from build123d import *

# Parameters (mm, degrees)
SKETCH_5_R = 7.5


with BuildPart() as part:
    # По траектории3: sweep along a path in Эскиз4
    with BuildLine(Plane.XY) as sweep_3_path:
        Line((-180, -170), (-120, -170))
        ThreePointArc((-120, -170), (-70.502525317, -149.497474683), (-50, -100))
        Line((-50, -100), (-50, -50))
        ThreePointArc((-50, -50), (-35.355339059, -14.644660941), (0, 0))
    # Эскиз5 → По траектории3 (sweep)
    with BuildSketch(Plane(origin=(0, 0, 0), x_dir=(0, 0, -1), z_dir=(1, 0, 0))):
        Circle(SKETCH_5_R)
    sweep_3 = sweep(path=sweep_3_path.line)

    # Зеркальное отражение4: По траектории3 across plane
    add(sweep_3.mirror(Plane(origin=(0, 0, 0), x_dir=(0, 0, 1), z_dir=(1, 0, 0))))


solid = part.part
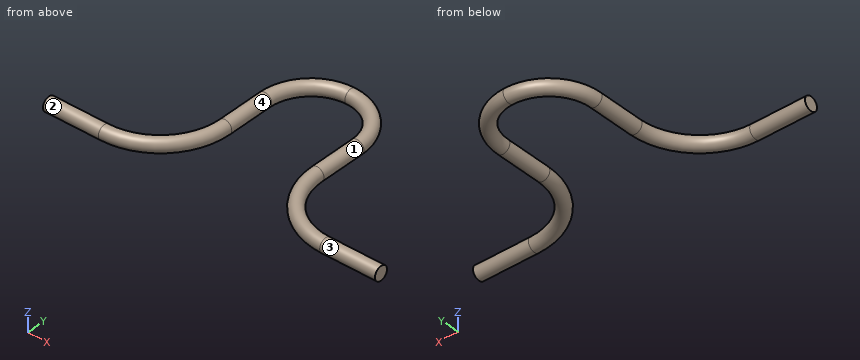
Can you work these out from the model? Positions are in its coordinate system, mm. Face numbers are marked on the shaded views. A direction names the side the tool comes from. Round coordinates to 2 decimals unless told otherwise and drop trailing zeros. Loops run counter-clockwise (first coordinate to the right, second up) from the corner with the lowest first, then second, coordinate; pieces in that order, holes last. Notation, with made-up numbers: (-23.75, 23) - (-13.75, 23) arc R24 cw to (-13.75, 39) - close; hole circle Ø9 at (-9.75, 18.25). An arc over 180 degrees is marked (long way). Answer in a Markdown table with one row per item. Add a question column.
Q1. We'd pull the mould along X, two halves only. Please class the marked faces 1 and 2: pulls with the +X half, pulls with the -X half, needs draft (parallel to the pull), parting line crosses it, or undercut.
Q2. I need wall thicknesses on L1, parallel to X at y = -52, z = 1; L2, parallel to X at y = -12, z = -0.5; L3, parallel to Y at x = -136, z = -0.5. Which ranges of each line are inside material? Lowest first, please.
Q3. I want a section at B-B on y = -66. List the corners of the cut face in (x, z) for me, and give its area (3 significant figures).
Q4. Which directions (+Z, -Z, +X, -X, +Y, -Y) give clear straight access to the entire face, cutting with the end or side of a thin tool? Please do the marked faces 3 and 4.
Q5. For pin 1 Ø5 at (y, z) = (-43.5, 5.5) entering from +X; pin 2 Ø3 at (x, z) = (79, -4.5) entering from -Y; pin 3 Ø1 at (x, z) = (-116, 1) entering from +Y, each with a flat end and sliding along its axis, tell me the tip position at first contact or that it passes through.
Q6. I want a section at A-A on z = 0. List the corners of the cut face in (x, y) for me.
Q7. I want a section at C-C on x = -131. List the corners of the cut face in (y, z) for me.
A:
| question | item | result |
|---|---|---|
| 1 | face 1 | undercut |
| 1 | face 2 | needs draft |
| 2 | L1 | -57.43 to -42.57, 42.57 to 57.43 |
| 2 | L2 | -43.13 to -19.07, 19.07 to 43.13 |
| 2 | L3 | -177.48 to -162.52 |
| 3 | outline | circle Ø15 at (-50, 0); circle Ø15 at (50, 0) |
| 3 | area | 353 mm^2 |
| 4 | face 3 | +X |
| 4 | face 4 | none |
| 5 | pin 1 | x = 56.53 |
| 5 | pin 2 | y = -165.44 |
| 5 | pin 3 | y = -162.38 |
| 6 | outline | (-180, -177.5) - (-120, -177.5) arc R77.5 ccw to (-42.5, -100) - (-42.5, -50) arc R42.5 cw to (42.5, -50) - (42.5, -100) arc R77.5 ccw to (120, -177.5) - (180, -177.5) - (180, -162.5) - (120, -162.5) arc R62.5 cw to (57.5, -100) - (57.5, -50) arc R57.5 ccw to (-57.5, -50) - (-57.5, -100) arc R62.5 cw to (-120, -162.5) - (-180, -162.5) - close |
| 7 | outline | circle Ø15 at (-170, 0) |
